from build123d import *

# Parameters (mm, degrees)
BOSS_EXTRUDE1_DEPTH  = 50
SKETCH2_R            = 1.6
CUT_EXTRUDE1_DEPTH   = 20
SKETCH4_W            = 4
SKETCH4_H            = 8
CUT_EXTRUDE2_DEPTH   = 12
BOSS_EXTRUDE4_DEPTH  = 7
BOSS_EXTRUDE12_DEPTH = 12.57
BOSS_EXTRUDE13_DEPTH = 12.57


with BuildPart() as part:
    # Sketch1 → Boss-Extrude1 (new body)
    with BuildSketch(Plane(origin=(0, 0, 0), x_dir=(1, 0, 0), z_dir=(0, 1, 0))):
        with BuildLine():
            Line((0, 0), (20, 0))
            Line((20, 0), (20, -24.855700299))
            ThreePointArc((20, -24.855700299), (19.469946725, -27.31925094), (17.973595405, -29.34680389))
            add(Edge.make_bspline(
                [(17.973595405, -29.34680389), (16.281120611, -30.60167495), (11.87635292, -29.319904822), (9.598231396, -25.56159513), (8.550503583, -23.49231552)],
                knots=[0, 0, 0, 0, 0.430742711, 1, 1, 1, 1], degree=3))
            Line((8.550503583, -23.49231552), (0, 0))
        make_face()
    extrude(amount=BOSS_EXTRUDE1_DEPTH)

    # Sketch2 → Cut-Extrude1 (cut)
    with BuildSketch(Plane(origin=(0, 0, 0), x_dir=(-1, 0, 0), z_dir=(0, 0, -1))):
        with Locations((-14, 31)):
            Circle(SKETCH2_R)
        with Locations((-14, 19)):
            Circle(SKETCH2_R)
    extrude(amount=-CUT_EXTRUDE1_DEPTH, mode=Mode.SUBTRACT)

    # Sketch4 → Cut-Extrude2 (cut)
    with BuildSketch(Plane(origin=(20, 0, 0), x_dir=(0, 0, -1), z_dir=(1, 0, 0))):
        with Locations((-9, 19)):
            Rectangle(SKETCH4_W, SKETCH4_H)
        with Locations((-9, 31)):
            Rectangle(SKETCH4_W, SKETCH4_H)
    extrude(amount=-CUT_EXTRUDE2_DEPTH, mode=Mode.SUBTRACT)

    # Sketch5 → Boss-Extrude4 (add)
    with BuildSketch(Plane(origin=(0, 0, 0), x_dir=(-1, 0, 0), z_dir=(0, 0, -1))):
        Polygon((-11.369100365, 37.428714266), (-12.760831375, 47.331394953), (-13.135879356, 50), (0, 50), (0, 37.428714266), align=None)
        Polygon((0, 12.571285734), (-11.369100365, 12.571285734), (-12.760831375, 2.668605047), (-13.135879356, 0), (0, 0), align=None)
    extrude(amount=BOSS_EXTRUDE4_DEPTH)

    # Sketch7 → Boss-Extrude12 (add)
    with BuildSketch(Plane(origin=(0, 50, 0), x_dir=(1, 0, 0), z_dir=(0, 1, 0))):
        Polygon((0, 0), (0, 7), (-2.54779164, 7), align=None)
    extrude(amount=-BOSS_EXTRUDE12_DEPTH)

    # Sketch8 → Boss-Extrude13 (add)
    with BuildSketch(Plane(origin=(0, 0, 0), x_dir=(-1, 0, 0), z_dir=(0, -1, 0))):
        Polygon((0, 0), (2.54779164, 7), (0, 7), align=None)
    extrude(amount=-BOSS_EXTRUDE13_DEPTH)


solid = part.part
Model file for the job. Use its own axes, mm. A direction names the side the tool comes from. Give positions to 0.01 mm unless a question says otherwise; leave off trailing zeros. Loops run counter-clockwise (first coordinate to the right, second up) from the corner with the lowest first, then second, coordinate; pieces in that order, holes last. Notation, with made-up numbers: (41.25, 52) - (51.25, 52) arc R29 cw to (51.25, 77) - close; hole circle Ø11 at (-3.75, 37). An arc over 180 degrees is marked (long way). Use one line per item in the form item = value.
(1) Drill centre lines: L1, parallel to Y at x = 13, z = 9; L2, parallel to Y at x = 14, z = 17.5; L3, parallel to Z at x = 16, y = 17.5. Where is each one in solid material? Low to high.
Determined:
L1 = 0 to 15, 23 to 27, 35 to 50
L2 = 0 to 17.4, 20.6 to 29.4, 32.6 to 50
L3 = 0 to 7, 11 to 30.07
(2) Cut at D-D (x = 17). Count the separate pieces of the cut face and the enclosed holes in it, then the cut area to 3 significant figures.
Determined:
separate_pieces = 1
enclosed_holes = 2
area = 1,430 mm^2
(3) Drop flat-ended pins along their axis: P1, Ø3.5, axis at x = 14, y = 32, coming from the -Z side; P2, Ø1.5, axis at x = 11, y = 29, coming from the +Z side; P3, Ø3, axis at y = 17.5, z = 9, coming from the +X side. Give the stop position or say it passes through.
Determined:
P1 = 0
P2 = 28.13
P3 = 8
(4) 3-axis set-ups, long thin cutter, end or side, ignore diameter. For faces 1 (the face through (6, 12.571, -3)), 2 (the face through (-1, 12.57, -4)), 3 (the face through (14, 15, 9)), 4 (the face through (12, 25, 0)): which of +Z, -Z, +X, -X, +Y, -Y reach the whole face in a straight line?
Determined:
face_1 = -Z, +X, -X
face_2 = +Z, -Z, +X, -X
face_3 = +X
face_4 = -Z, +X
(5) Pull direction Y, two halves, no side cores. Call faces 5 (the face through (11, 0, 12)), 6 (the face through (14, 21, 7)), 7 (the face through (5, 6, -7)): pulls with the +Y half, pulls with the -Y half, needs draft (parallel to the pull), parting line crosses it, or undercut.
Determined:
face_5 = pulls with the -Y half
face_6 = undercut
face_7 = needs draft
(6) Cut at C-C (x = 7.25). Give the cut face in (y, z).
Determined:
outline = (0, -7) - (12.57, -7) - (12.57, 0) - (37.43, 0) - (37.43, -7) - (50, -7) - (50, 19.92) - (0, 19.92) - close
(7) Cut at A-A (z = 16). Give the cut face in (x, y).
Determined:
outline = (5.82, 0) - (20, 0) - (20, 50) - (5.82, 50) - close; hole circle Ø3.2 at (14, 19); hole circle Ø3.2 at (14, 31)
(8) Cut at B-B (z = 9). Give the cut face in (x, y).
Determined:
outline = (3.28, 0) - (20, 0) - (20, 15) - (8, 15) - (8, 23) - (20, 23) - (20, 27) - (8, 27) - (8, 35) - (20, 35) - (20, 50) - (3.28, 50) - close
